Autodesk Inventor part; units mm, degrees
ref_plane "YZ Plane" through (0, 0, 0) normal (1, 0, 0) x (0, 1, 0)
ref_plane "XZ Plane" through (0, 0, 0) normal (0, 1, 0) x (-1, 0, 0)
ref_plane "XY Plane" through (0, 0, 0) normal (0, 0, 1) x (1, 0, 0)
sketch "MainSketch" plane through (0, 0, 0) normal (0, 1, 0) x (-1, 0, 0)
  line L0 (31, -50) -> (-31, -50)
  line L1 (-31, -50) -> (-31, 50)
  line L2 (-31, 50) -> (31, 50)
  line L3 (31, 50) -> (31, -50)
  line L4 (31, -49.4494) -> (-31, 50.5506) construction
  line L5 (-31, -50) -> (31, 50) construction
  line L6 (31, 50) -> (-31, 50)
  line L7 (-31, 50) -> (-31, 21.5)
  line L8 (-31, 21.5) -> (31, 21.5)
  line L9 (31, 21.5) -> (31, 50)
  line L10 (-31, -50) -> (16, -50)
  line L11 (16, -50) -> (16, 21.5)
  line L12 (16, 21.5) -> (-31, 21.5)
  line L13 (-31, 21.5) -> (-31, -50)
  line L14 (31, 21.5) -> (16, 21.5)
  line L15 (16, 21.5) -> (16, -50)
  line L16 (16, -50) -> (31, -50)
  line L17 (31, -50) -> (31, 21.5)
  line L18 (-31, 21.5) -> (-31, 35.75)
  line L19 (-31, 21.5) -> (-31, 35.75)
  arc A0 (0, 50) -> (-31, 21.5) centre (0.8091, 18.0102) ccw
  line L20 (29.5, 48.5) -> (-29.5, 48.5)
  line L21 (-29.5, 48.5) -> (-29.5, -48.5)
  line L22 (-29.5, -48.5) -> (29.5, -48.5)
  line L23 (29.5, -48.5) -> (29.5, 48.5)
  line L24 (29.5, 48.5) -> (-29.5, -48.5) construction
  line L25 (-29.5, 48.5) -> (29.5, -48.5) construction
  line L26 (-29.5, -48.5) -> (16, -48.5)
  line L27 (16, -48.5) -> (16, 2.2597)
  line L28 (16, 2.2597) -> (-29.5, 2.2597)
  line L29 (-29.5, 2.2597) -> (-29.5, -48.5)
  line L30 (16, -48.5) -> (29.5, -48.5)
  line L31 (29.5, -48.5) -> (29.5, 11.5)
  line L32 (29.5, 11.5) -> (16, 11.5)
  line L33 (16, 11.5) -> (16, -48.5)
  line L34 (29.5, 21.5) -> (16, 21.5)
  line L35 (16, 21.5) -> (16, 11.5)
  line L36 (16, 11.5) -> (29.5, 11.5)
  line L37 (29.5, 11.5) -> (29.5, 21.5)
  line L38 (29.5, 21.5) -> (29.5, 11.5)
  line L39 (29.5, 16.5) -> (16, 16.5)
  line L40 (22.75, 16.5) -> (22.75, 11.5)
  line L41 (22.75, 16.5) -> (22.75, 21.5)
  circle A1 centre (22.75, 16.5) radius 4
  arc A2 (0, 48.5) -> (-29.5, 21.5) centre (0.9166, 17.8828) ccw
  line L42 (-20.0675, 15.4609) -> (-7.0675, 15.4609)
  line L43 (-7.0675, 15.4609) -> (-7.0675, -23.5689)
  line L44 (-7.0675, -23.5689) -> (-20.0675, -23.5689)
  line L45 (-20.0675, -23.5689) -> (-20.0675, 15.4609)
  line L46 (22.75, 11.5) -> (22.75, -28.5)
  line L47 (22.75, 11.5) -> (62.75, 11.5) construction
  line L48 (20.2505, -33.5) -> (20.2505, -28.5)
  line L49 (22.75, -28.5) -> (25.2505, -28.5)
  line L50 (20.2505, -28.5) -> (25.2505, -28.5)
  line L51 (25.2505, -28.5) -> (25.2505, -33.5)
  line L52 (25.2505, -33.5) -> (20.2505, -33.5)
  line L53 (20.2505, -33.5) -> (20.2505, -28.5)
  line L54 (25.2505, -28.5) -> (20.2505, -33.5)
  line L55 (20.2505, -28.5) -> (25.2505, -33.5)
  circle A3 centre (22.7505, -31) radius 5
  line L56 (-7.0675, 15.4609) -> (-20.0675, 15.4609)
  line L57 (-20.0675, 15.4609) -> (-20.0675, 10.4609)
  line L58 (-20.0675, 10.4609) -> (-7.0675, 10.4609)
  line L59 (-7.0675, 10.4609) -> (-7.0675, 15.4609)
  line L60 (-7.0675, -23.5689) -> (-20.0675, -23.5689)
  line L61 (-20.0675, -23.5689) -> (-20.0675, -18.5689)
  line L62 (-20.0675, -18.5689) -> (-7.0675, -18.5689)
  line L63 (-7.0675, -18.5689) -> (-7.0675, -23.5689)
  line L64 (-29.5, -48.5) -> (-16.5, -48.5)
  line L65 (-16.5, -48.5) -> (-8.5, -48.5)
  line L66 (-8.5, -48.5) -> (-8.5, -42.5)
  line L67 (-8.5, -42.5) -> (-16.5, -42.5)
  line L68 (-16.5, -42.5) -> (-16.5, -48.5)
  line L69 (-8.5, -42.5) -> (-4.5, -42.5)
  line L70 (-8.5, -42.5) -> (-4.5, -42.5) construction
  line L71 (-4.5, -42.5) -> (-3.5, -42.5)
  line L72 (-3.5, -42.5) -> (-3.5, -40.5)
  line L73 (-3.5, -40.5) -> (-4.5, -40.5)
  line L74 (-4.5, -40.5) -> (-4.5, -42.5)
  line L75 (-4.5, -42.5) -> (-3.5, -42.5)
  line L76 (-3.5, -42.5) -> (-3.5, -44.5)
  line L77 (-3.5, -44.5) -> (-4.5, -44.5)
  line L78 (-4.5, -44.5) -> (-4.5, -42.5)
  line L79 (-8.5, -42.5) -> (-8.5, -10.5)
  line L80 (-8.5, -10.5) -> (-10.5, -10.5)
  line L81 (-10.5, -10.5) -> (-10.5, -9.5)
  line L82 (-10.5, -9.5) -> (-8.5, -9.5)
  line L83 (-8.5, -9.5) -> (-8.5, -10.5)
  line L84 (-8.5, -42.5) -> (-8.5, -37.5)
  line L85 (-8.5, -37.5) -> (-9.5, -37.5)
  line L86 (-9.5, -37.5) -> (-9.5, -39.5)
  line L87 (-9.5, -39.5) -> (-8.5, -39.5)
  line L88 (-8.5, -39.5) -> (-8.5, -37.5)
  point P0 (0, 0)
  dimension "d0" = 62
  dimension "d1" = 100
  dimension "d2" = 62
  dimension "d3" = 28.5
  dimension "d4" = 47
  dimension "d5" = 32
  dimension "d6" = 59
  dimension "d7" = 97
  dimension "d8" = 60
  dimension "d9" = 8
  dimension "d10" = 39.0299
  dimension "d11" = 13
  dimension "d12" = 40
  dimension "d13" = 90
  dimension "d14" = 5
  dimension "d15" = 5
  dimension "d16" = 10
  dimension "d17" = 5
  dimension "d18" = 5
  dimension "d19" = 13
  dimension "d20" = 8
  dimension "d21" = 6
  dimension "d22" = 4
  dimension "d23" = 0
  dimension "d24" = 1
  dimension "d25" = 2
  dimension "d26" = 2
  dimension "d27" = 32
  dimension "d28" = 2
  dimension "d29" = 1
  dimension "d30" = 5
  dimension "d31" = 1
  dimension "d32" = 2
extrude "MainExtrusion" add sketch "MainSketch" along normal blind 6 contours L49 L54 L55 L50 | A3 | L51 L55 L54 | L55 L54 L48 | L52 L54 L55
sketch "ButtonBlockerSketch" plane through (-22.7505, 0, -31) normal (0, -1, 0) x (1, 0, 0)
  circle A0 centre (0, 0) radius 6
  point P0 (22.7505, 31)
  dimension "d35" = 12
extrude "ButtonBlockerExtrusion" add sketch "ButtonBlockerSketch" against normal blind 1
fillet "MainConnection" radius 3 1 edges at (-17.7505, 6, -31)
sketch "ClickerProtusionSketch" plane through (-22.7505, 0, -31) normal (0, -1, 0) x (1, 0, 0)
  line L0 (2.5, 2.5) -> (-2.5, 2.5)
  line L1 (-2.5, 2.5) -> (-2.5, -2.5)
  line L2 (-2.5, -2.5) -> (2.5, -2.5)
  line L3 (2.5, -2.5) -> (2.5, 2.5)
  line L4 (2.5, 2.5) -> (-2.5, -2.5) construction
  line L5 (-2.5, 2.5) -> (2.5, -2.5) construction
  point P0 (22.7505, 31)
  point P1 (0, 0)
  dimension "d39" = 5
  dimension "d40" = 5
extrude "ClickerProtusionExtrusion" add sketch "ClickerProtusionSketch" along normal blind 23
fillet "ClickerProtusionConnection" radius 1 4 edges at (-20.2505, -11.5, -33.5) (-20.2505, -11.5, -28.5) (-25.2505, -11.5, -33.5) (-25.2505, -11.5, -28.5)
properties part number "EvoTest_body"
Model file for the job. Use its own axes, mm. A direction names the side the tool comes from. Coordinates: 2 decimals unless noted, no trailing zeros. Loops run counter-clockwise (first coordinate to the right, second up) from the corner with the lowest first, then second, coordinate; pieces in that order, holes last. Notation, with made-up numbers: (69, 3.5) - (125, 3.5) arc R15 cw to (125, 18.5) - close; hole circle Ø3 at (-40, 74.25). An arc over 180 degrees is marked (long way). Answer as a JSON object with one key per item and string values. Group by question number.
(1) Flat gauge pins, fed straight in: pin 1 (2 mm diameter, centred on x = -25, y = -3.5, fed in from -Z); pin 2 (3 mm diameter, centred on x = -18, y = -6.5, fed in from +Z); pin 3 (1 mm diameter, centred on y = -1, z = -29, fed in from -X); pin 4 (0.9 mm diameter, centred on x = -22, y = -13.5, fed in from +Z). Where does each tip first touch, or does it go through?
(2) Cut at A-A (y = -9.75). Give the cut face in (x, z).
(3) Probe line 1 along X through (y, z) = (-6.75, -29.5); line 2 along Y through (x, z) = (-24.75, -35.75); line 3 along Z through (x, y) = (-22.25, -6.5). List the from-to ranges inside material, lowest first.
(4) Tool access for faces 1 (the face through (-23, -11, -28.5)), 2 (the face through (-20.551, -11.661, -33.215)), 3 (the face through (-25.058, 1.986, -26.564)), 4 (the face through (-20.25, -11, -31)): list every direction of +Z, -Z, +X, -X, +Y, -Y with a clear straight run to the whole face (end or side of a thin tool).
Geometry says:
{
 "1": {"pin 1": "stops at z = -33.5", "pin 2": "passes through", "pin 3": "stops at x = -25.25", "pin 4": "stops at z = -28.5"},
 "2": {"outline": "(-25.25, -32.5) arc R1 ccw to (-24.25, -33.5) - (-21.25, -33.5) arc R1 ccw to (-20.25, -32.5) - (-20.25, -29.5) arc R1 ccw to (-21.25, -28.5) - (-24.25, -28.5) arc R1 ccw to (-25.25, -29.5) - close"},
 "3": {"line 1": "x = -25.25 to -20.25", "line 2": "y = 0 to 1", "line 3": "z = -33.5 to -28.5"},
 "4": {"face 1": "+Z, +X, -X, -Y", "face 2": "-Z, +X, -Y", "face 3": "+Y", "face 4": "+Z, -Z, +X, -Y"}
}
